Geometry check sheet. Reference: the model listing, model coordinates, mm. Face numbers are marked on the shaded views. A direction names the side the tool comes from. Round coordinates to 2 decimals unless told otherwise and drop trailing zeros. Write each loop counter-clockwise with the first axis right and the second up, starting at its lowest first coordinate (ties: lowest second). Pieces come first, ordered by that corner, then holes. Notation, with made-up numbers: M 50.5,66 L 64.5,66 A13 ccw 64.5,84 Z; hole C 64,82 d1. An arc over 180 degrees is marked long. One line per item, written item: value. Start each with the question number.
1. Access from +Z, -Z, +X, -X, +Y, -Y to the whole of each face (thin tool, end or side, straight path). Record for the marked faces 4, 5, 6, 7 and 8.
2. Section check C-C (x = 42.5). Record the boundary of the cut face in (y, z).
3. Release check for a two-part mould opening along X. For the marked faces 1, 2 and 3 record: pulls with the +X half, pulls with the -X half, needs draft (parallel to the pull), parting line crosses it, or undercut.
4. Section check B-B (z = 21). Record the boundary of the cut face in (x, y).
5. Section check A-A (y = -18.25). Record the boundary of the cut face in (x, z).
6. Depth check by flat-ended pin: P1, Ø8, axis at y = -15, z = -19.5, coming from the +X side; P2, Ø3, axis at x = 37.5, y = -15.5, coming from the -Z side; P3, Ø10, axis at x = -4.5, y = -11, coming from the +Z side. Enter the tip coordinate at first touch or a pass-through.
7. Scan lines: probe 1 along X at (y, z) = (-15, 16.5); probe 2 along X at (y, z) = (-13.75, -37); probe 3 along X at (y, z) = (-13.75, 38.5). Record each from-to range of solid material in increasing order. Write a range as [from, to].
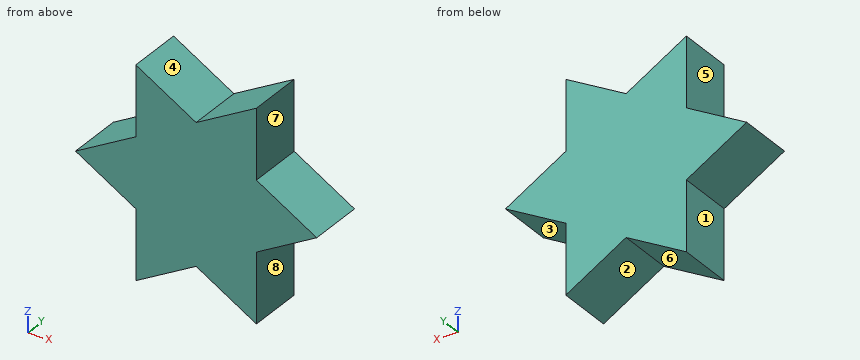
from build123d import *

# Parameters (mm, degrees)
F1_DEPTH = 25.4


with BuildPart() as f1:
    # F0 (on Front) → F1 (new body)
    with BuildSketch(Plane.XZ):
        Polygon((27.7888969147, 48.1317813425), (0, 32.0878542283), (27.7888969147, 16.0439271142), align=None)
        Polygon((27.7888969147, 16.0439271142), (0, 32.0878542283), (-27.7888969147, 16.0439271142), (-27.7888969147, -16.0439271142), (0, -32.0878542283), (27.7888969147, -16.0439271142), align=None)
        Polygon((-27.7888969147, 16.0439271142), (0, 32.0878542283), (-27.7888969147, 48.1317813425), align=None)
        Polygon((55.5777938294, 0), (27.7888969147, 16.0439271142), (27.7888969147, -16.0439271142), align=None)
        Polygon((-27.7888969147, -16.0439271142), (-27.7888969147, 16.0439271142), (-55.5777938294, 0), align=None)
        Polygon((27.7888969147, -48.1317813425), (27.7888969147, -16.0439271142), (0, -32.0878542283), align=None)
        Polygon((0, -32.0878542283), (-27.7888969147, -16.0439271142), (-27.7888969147, -48.1317813425), align=None)
    extrude(amount=F1_DEPTH)


solid = f1.part
Result sheet:
1. face 4: +Z, +Y, -Y
1. face 5: +Z, -X, +Y, -Y
1. face 6: -Z, +Y, -Y
1. face 7: +Z, +X, +Y, -Y
1. face 8: -Z, +X, +Y, -Y
2. outline: M -25.4,-7.55 L 0,-7.55 L 0,7.55 L -25.4,7.55 Z
3. face 1: pulls with the -X half
3. face 2: undercut
3. face 3: pulls with the +X half
4. outline: M -27.79,-25.4 L 27.79,-25.4 L 27.79,0 L -27.79,0 Z
5. outline: M -55.58,0 L -27.79,-16.04 L -27.79,-48.13 L 0,-32.09 L 27.79,-48.13 L 27.79,-16.04 L 55.58,0 L 27.79,16.04 L 27.79,48.13 L 0,32.09 L -27.79,48.13 L -27.79,16.04 Z
6. P1: stops at x = 28.73
6. P2: stops at z = -11.3
6. P3: stops at z = 37.57
7. probe 1: x = [-27.79, 27.79]
7. probe 2: x = [-27.79, -8.51], [8.51, 27.79]
7. probe 3: x = [-27.79, -11.11], [11.11, 27.79]
